```python
from build123d import *

# Parameters (mm, degrees)
F0_R     = 6.35
F1_DEPTH = 5.08
F2_R     = 2.53999
F3_R     = 0.762
F4_DEPTH = 0.254


# Not quite as in the source:
# - a fillet or chamfer is up to 0.001 mm smaller than in the source, because OpenCascade refuses the exact size


with BuildPart() as f1:
    # F0 (on Right) → F1 (new body)
    with BuildSketch(Plane.YZ):
        Circle(F0_R)
    extrude(amount=F1_DEPTH)

    # F2 (radius 2.54 in the source; OpenCascade refuses exactly that, so slightly less here)
    f2_edges = [f1.edges().sort_by_distance(p)[0] for p in [
        (5.08, -6.35, 0),
        (0, -6.35, 0),
    ]]
    fillet(f2_edges, radius=F2_R)

    # F3 (on face) → F4 (cut)
    with BuildSketch(Plane.YZ.offset(5.08)):
        Circle(F3_R)
    extrude(amount=-F4_DEPTH, mode=Mode.SUBTRACT)


solid = f1.part
```
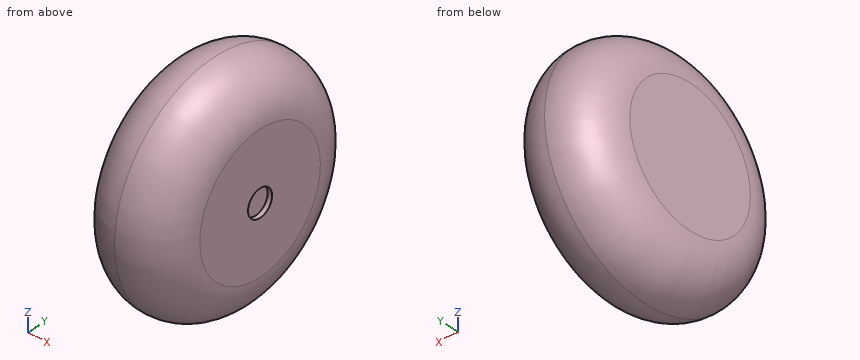
Geometry check sheet. Reference: the model listing, model coordinates, mm. Coordinates: 2 decimals unless noted, no trailing zeros. Order: outer loops, then holes, each group sorted by start corner. A loop starts at its lowest first (then second) coordinate and runs counter-clockwise, first axis right, second up. Notation, with made-up numbers: (31.25, 54.25) - (50.25, 54.25) arc R14 cw to (50.25, 78.25) - close; hole circle Ø3 at (80.5, 82). An arc over 180 degrees is marked (long way). Use one line per item in the form item = value.
1. Section check D-D (x = 1.4). Record the boundary of the cut face in (y, z).
Here are the results:
outline = circle Ø12.16 at (0, 0)
2. Gauge pin test, flat ends, axial feed: pin 1 (1.2 mm diameter, centred on y = 0.5, z = 0, fed in from +X); pin 2 (2 mm diameter, centred on x = 2, y = -4.5, fed in from -Z); pin 3 (1.5 mm diameter, centred on x = 1, z = 0, fed in from -Y); pin 4 (0.9 mm diameter, centred on y = 0, z = 0, fed in from +X). Record the tip position at first contact, or that the pin passes through.
Here are the results:
pin_1 = 5.08
pin_2 = -5.26
pin_3 = -6.22
pin_4 = 4.83
3. Scan lines: line 1 (Y direction, x = 1.85, z = 1.25); line 2 (X direction, y = -5.25, z = -1.5); line 3 (Z direction, x = 4.15, y = -1.5). Record each from-to range of solid material in increasing order.
Here are the results:
line_1 = -6.13 to 6.13
line_2 = 0.61 to 4.47
line_3 = -5.58 to 5.58
4. Section check C-C (x = 0.35). Record the boundary of the cut face in (y, z).
Here are the results:
outline = circle Ø10.19 at (0, 0)
